from build123d import *

# Parameters (mm, degrees)
EXTRUDE_7_DEPTH                = 7
SKETCH_3_W                     = 102
SKETCH_3_H                     = 63.98
CUT_EXTRUDE_5_DEPTH            = 5
SKETCH_11_R                    = 4.77
EXTRUDE_8_DEPTH                = 40
HOLE_WIZARD_M3_5_2_D           = 2.9
HOLE_WIZARD_M3_5_2_DEPTH       = 10
HOLE_WIZARD_M3_5_2_CSINK_D     = 3.55
HOLE_WIZARD_M3_5_2_CSINK_ANGLE = 90
HOLE_WIZARD_M3_5_2_TIP         = 0.871247898


with BuildPart() as part:
    # 草图1 → 凸台-拉伸7 (new body)
    with BuildSketch(Plane(origin=(0, 0, 0), x_dir=(1, 0, 0), z_dir=(0, 1, 0))):
        Polygon((0, 64), (0, 79), (102, 79), (102, 64), (107, 64), (107, 0), (102, 0), (102, -15), (0, -15), (0, 0), (-5, 0), (-5, 64), align=None)
    extrude(amount=EXTRUDE_7_DEPTH)

    # 草图3 → 切除-拉伸5 (cut)
    with BuildSketch(Plane(origin=(0, 7, 0), x_dir=(1, 0, 0), z_dir=(0, 1, 0))):
        with Locations((51, 32)):
            Rectangle(SKETCH_3_W, SKETCH_3_H)
    extrude(amount=-CUT_EXTRUDE_5_DEPTH, mode=Mode.SUBTRACT)

    # 草图11 → 凸台-拉伸8 (add)
    with BuildSketch(Plane(origin=(0, 7, 0), x_dir=(1, 0, 0), z_dir=(0, 1, 0))):
        with Locations(Location((35, 70.4, 0), (0, 0, 270))):
            Circle(SKETCH_11_R)
        with Locations(Location((94.484841374, 70.4, 0), (0, 0, 270))):
            Circle(SKETCH_11_R)
        with Locations(Location((94.484841374, -6.4, 0), (0, 0, 90))):
            Circle(SKETCH_11_R)
        with Locations(Location((35, -6.4, 0), (0, 0, 90))):
            Circle(SKETCH_11_R)
    extrude(amount=EXTRUDE_8_DEPTH)

    # M3.5 螺纹孔2
    with Locations(Plane(origin=(35, 47, -70.4), x_dir=(0, 0, 1), z_dir=(0, 1, 0))):
        with Locations((0, 0), (0, 59.484841374), (76.8, 59.484841374), (76.8, 0)):
            CounterSinkHole(HOLE_WIZARD_M3_5_2_D / 2, HOLE_WIZARD_M3_5_2_CSINK_D / 2, depth=HOLE_WIZARD_M3_5_2_DEPTH, counter_sink_angle=HOLE_WIZARD_M3_5_2_CSINK_ANGLE)
            with Locations((0, 0, -(HOLE_WIZARD_M3_5_2_DEPTH + HOLE_WIZARD_M3_5_2_TIP / 2))):  # 118° drill point
                Cone(0, HOLE_WIZARD_M3_5_2_D / 2, HOLE_WIZARD_M3_5_2_TIP, mode=Mode.SUBTRACT)


solid = part.part
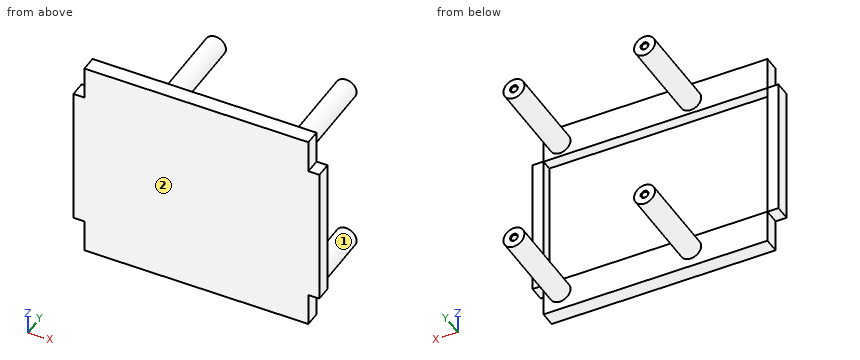
Model file for the job. Use its own axes, mm. Face numbers are marked on the shaded views. Coordinates: 2 decimals unless noted, no trailing zeros. Order: outer loops, then holes, each group sorted by start corner. A loop starts at its lowest first (then second) coordinate and runs counter-clockwise, first axis right, second up. Notation, with made-up numbers: (-12, 71) -> (-6, 71) arc R32 cw to (-6, 110) -> close; hole circle Ø6 at (53, 38). An arc over 180 degrees is marked (long way). Return JSON: item names as keys, results as strings. Group by question number.
Item 1: Saw through at B-B on y = 14.5. Write the cut outline in (x, z), then the cut area to 3 significant figures.
Item 2: Flat gauge pins, fed straight in: P1, Ø2.5, axis at x = 94.48, z = 6.4, coming from the -Y side; P2, Ø10, axis at x = 44, z = -3.5, coming from the +Y side; P3, Ø4, axis at y = 28, z = 2.5, coming from the +X side; P4, Ø2.5, axis at x = 35, z = 6.4, coming from the +Y side. Where does each tip first touch, or does it go through?
Item 3: Pull direction X, two halves, no side cores. Call the marked faces 1 and 2: pulls with the +X half, pulls with the -X half, needs draft (parallel to the pull), parting line crosses it, or undercut.
Item 4: Saw through at A-A on z = -3. Write the cut outline in (x, y).
Item 5: Wall check: line 1 along X through (y, z) = (42, -70.4); line 2 along X through (y, z) = (39, -70); line 3 along X through (y, z) = (2.5, -31). Give the ranges that are in metal, low to high. Write a range as [from, to].
Values found:
{
 "1": {"outline": "circle Ø9.54 at (35, -70.4); circle Ø9.54 at (35, 6.4); circle Ø9.54 at (94.48, -70.4); circle Ø9.54 at (94.48, 6.4)", "area": "286 mm2"},
 "2": {"P1": "stops at y = 0", "P2": "stops at y = 7", "P3": "stops at x = 98.86", "P4": "stops at y = 36.88"},
 "3": {"face 1": "undercut", "face 2": "needs draft"},
 "4": {"outline": "(-5, 0) -> (107, 0) -> (107, 7) -> (102, 7) -> (102, 2) -> (0, 2) -> (0, 7) -> (-5, 7) -> close"},
 "5": {"line 1": "x = [30.23, 33.55], [36.45, 39.77], [89.71, 93.03], [95.93, 99.25]", "line 2": "x = [30.25, 33.61], [36.39, 39.75], [89.73, 93.09], [95.88, 99.24]", "line 3": "x = [-5, 0], [102, 107]"}
}
